The listing builds one solid part. Answer for the finished solid, in the listing's coordinates (mm). Face numbers are marked on the shaded views. A direction names the side the tool comes from. Give positions to 0.01 mm unless a question says otherwise; leave off trailing zeros. Loops run counter-clockwise (first coordinate to the right, second up) from the corner with the lowest first, then second, coordinate; pieces in that order, holes last. Notation, with made-up numbers: (20, -2) - (59, -2) arc R22 cw to (59, 15) - close; hole circle Ø11 at (52, 65.25). An arc over 180 degrees is marked (long way). Write item = value, one per line. Start each with the question number.
1) The part is cut by section D-D on x = 16.5. Write down the section's boundary in (y, z), plus the area to 3 significant figures.
2) The part is cut by section A-A on x = 0. Write down the section's boundary in (y, z).
3) The part is cut by section C-C on y = 0. Write down the section's boundary in (x, z).
4) Which of the six approach directions +Z, -Z, +X, -X, +Y, -Y give full straight-line access (tool end or side, diameter ignored) to the marked faces 1, 2 and 3?
5) Consider probe 1 along X at (y, z) = (-29, 14); probe 2 along Y at (x, z) = (15.5, 6.3); probe 3 along Y at (x, z) = (-8, 39.5). Determine where each line is inside the solid, lowest interval first.
6) The part is cut by section B-B on z = 31. Write down the section's boundary in (x, y).
7) Flat-ended cylindrical pins translate along their axes: P1, Ø10, axis at x = 2.5, z = 25.5, coming from the +Y side; P2, Ø2.5, axis at x = 8, y = -8, coming from the +Z side; P3, Ø4, axis at x = -8, y = -8, coming from the +Z side; P4, Ø3.5, axis at x = -8.5, z = 31, coming from the +Y side. Find the tip coordinate at first contact, or state that the pin passes through.
8) The mould has two halves that part along Y. Classify the marked faces 4, 5 and 6: +Y half, -Y half, draft (parallel to the pull), parting line (faces both ways), or undercut.
from build123d import *

# Parameters (mm, degrees)
MOTOR_MOUNT_SOLID_DEPTH                   = 7.5
ENCODER_DISTANCE_SKETCH_W                 = 50
ENCODER_DISTANCE_SKETCH_H                 = 45
ENCODER_DISTANCE_SOLID_DEPTH              = 5
ENCODER_MOUNT_SKETCH_R                    = 1.45
ENCODER_MOUNT_SKETCH_W                    = 7
ENCODER_MOUNT_SKETCH_H                    = 9
ENCODER_MOUNT_SOLID_DEPTH                 = 5
MOTOR_CLAMP_MOUNTING_HOLES_CUT_DEPTH      = 78.661122835
MOTOR_CLAMP_MOUNTING_HOLES_CUT_DEPTH_BACK = 78.661122835
MOTOR_CLAMP_MOUNTING_HOLES_SKETCH_R       = 1.45
GUSSET_PLATE_SKETCH_W                     = 50
GUSSET_PLATE_SKETCH_H                     = 5
GUSSET_PLATE_SOLID_DEPTH                  = 16.5
GUSSET_SOLID_DEPTH                        = 1.5
MOUNTING_PLATE_SKETCH_W                   = 50
MOUNTING_PLATE_SKETCH_H                   = 92
MOUNTING_PLATE_SKETCH_R                   = 2.65
MOUNTING_PLATE_SOLID_DEPTH                = 5
MOUNTING_HOLES_CUT_DEPTH                  = 93.348524623
MOUNTING_HOLES_CUT_DEPTH_BACK             = 93.348524623
MOUNTING_HOLE_SKETCH_R                    = 2.65
MOUNTING_PLATE_TRIM_SKETCH_W              = 50
MOUNTING_PLATE_TRIM_SKETCH_H              = 25.5
MOUNTING_PLATE_TRIM_SKETCH_H_2            = 30
MOUNTING_PLATE_TRIM_SKETCH_W_2            = 23.5
MOUNTING_PLATE_TRIM_SKETCH_H_3            = 16.5
MOUNTING_PLATE_TRIM_CUT_DEPTH             = 2
CUT_EXTRUDE1_DEPTH                        = 93.990590922
CUT_EXTRUDE1_DEPTH_BACK                   = 93.990590922
SKETCH2_W                                 = 50
SKETCH2_H                                 = 120
SKETCH2_W_2                               = 42
SKETCH2_H_2                               = 54.272597004
SKETCH3_W                                 = 42
SKETCH3_H                                 = 59.586450004
BOSS_EXTRUDE1_DEPTH                       = 5
CUT_EXTRUDE2_DEPTH                        = 69.16716098
CUT_EXTRUDE2_DEPTH_BACK                   = 69.16716098
SKETCH4_R                                 = 2.15
SKETCH5_W                                 = 42
SKETCH5_H                                 = 42
BOSS_EXTRUDE2_DEPTH                       = 5
SKETCH6_W                                 = 42
SKETCH6_H                                 = 53.136298502
CUT_EXTRUDE3_DEPTH                        = 10
SKETCH7_R                                 = 12.5
SKETCH7_R_2                               = 1.7
CUT_EXTRUDE4_DEPTH                        = 5
SKETCH8_R                                 = 5
CUT_EXTRUDE5_DEPTH                        = 56.441335495


with BuildPart() as part:
    # Mouting Mount Sketch → Motor Mount Solid (new, symmetric)
    with BuildSketch(Plane.XY):
        with BuildLine():
            Line((-25, -55), (25, -55))
            Line((25, -55), (25, 0))
            Line((25, 0), (10, 0))
            ThreePointArc((10, 0), (0, -10), (-10, 0))
            Line((-10, 0), (-25, 0))
            Line((-25, 0), (-25, -55))
        make_face()
    extrude(amount=MOTOR_MOUNT_SOLID_DEPTH, both=True)

    # Encoder Distance Sketch → Encoder Distance Solid (add)
    with BuildSketch(Plane.XZ.offset(55)):
        with Locations((0, 15)):
            Rectangle(ENCODER_DISTANCE_SKETCH_W, ENCODER_DISTANCE_SKETCH_H)
    extrude(amount=ENCODER_DISTANCE_SOLID_DEPTH)

    # Encoder Mount Sketch → Encoder Mount Solid (add)
    with BuildSketch(Plane.XY.offset(37.5)):
        Polygon((-25, -60), (-25, -55), (-11.5, 11.5), (11.5, 11.5), (25, -55), (25, -60), align=None)
        with Locations((-8, 8)):
            Circle(ENCODER_MOUNT_SKETCH_R, mode=Mode.SUBTRACT)
        with Locations((8, 8)):
            Circle(ENCODER_MOUNT_SKETCH_R, mode=Mode.SUBTRACT)
        with Locations((-8, -8)):
            Circle(ENCODER_MOUNT_SKETCH_R, mode=Mode.SUBTRACT)
        with Locations((8, -8)):
            Circle(ENCODER_MOUNT_SKETCH_R, mode=Mode.SUBTRACT)
        with Locations((-8, 0)):
            Rectangle(ENCODER_MOUNT_SKETCH_W, ENCODER_MOUNT_SKETCH_H, mode=Mode.SUBTRACT)
        with Locations((8, 0)):
            Rectangle(ENCODER_MOUNT_SKETCH_W, ENCODER_MOUNT_SKETCH_H, mode=Mode.SUBTRACT)
    extrude(amount=ENCODER_MOUNT_SOLID_DEPTH)

    # Motor Clamp Mounting Holes Sketch → Motor Clamp Mounting Holes Cut (cut, two sides: drawn at the far end of the back side and taken through both)
    with BuildSketch(Plane(origin=(0, 0, 0), x_dir=(1, 0, 0), z_dir=(0, 1, 0)).offset(-MOTOR_CLAMP_MOUNTING_HOLES_CUT_DEPTH_BACK)):
        with Locations(Location((-15, 0, 0), (0, 0, 180))):
            Circle(MOTOR_CLAMP_MOUNTING_HOLES_SKETCH_R)
        with Locations(Location((15, 0, 0), (0, 0, 180))):
            Circle(MOTOR_CLAMP_MOUNTING_HOLES_SKETCH_R)
    extrude(amount=MOTOR_CLAMP_MOUNTING_HOLES_CUT_DEPTH + MOTOR_CLAMP_MOUNTING_HOLES_CUT_DEPTH_BACK, mode=Mode.SUBTRACT)

    # Gusset Plate Sketch → Gusset Plate Solid (add)
    with BuildSketch(Plane.XY.offset(42.5)):
        with Locations((0, -57.5)):
            Rectangle(GUSSET_PLATE_SKETCH_W, GUSSET_PLATE_SKETCH_H)
    extrude(amount=GUSSET_PLATE_SOLID_DEPTH)

    # Gusset Sketch → Gusset Solid (add, symmetric)
    with BuildSketch(Plane(origin=(0, 0, 0), x_dir=(0, 0, -1), z_dir=(1, 0, 0))):
        Polygon((-42.5, 11.5), (-59, -55), (-42.5, -55), align=None)
    extrude(amount=GUSSET_SOLID_DEPTH, both=True)

    # Mounting Plate Sketch → Mounting Plate Solid (add)
    with BuildSketch(Plane(origin=(0, -55, 0), x_dir=(1, 0, 0), z_dir=(0, 1, 0))):
        with Locations((0, -13)):
            Rectangle(MOUNTING_PLATE_SKETCH_W, MOUNTING_PLATE_SKETCH_H)
        with Locations((-19, -53)):
            Circle(MOUNTING_PLATE_SKETCH_R, mode=Mode.SUBTRACT)
        with Locations((19, -53)):
            Circle(MOUNTING_PLATE_SKETCH_R, mode=Mode.SUBTRACT)
        with Locations(Location((-19, 27, 0), (0, 0, 270))):
            Circle(MOUNTING_PLATE_SKETCH_R, mode=Mode.SUBTRACT)
        with Locations(Location((19, 27, 0), (0, 0, 270))):
            Circle(MOUNTING_PLATE_SKETCH_R, mode=Mode.SUBTRACT)
    extrude(amount=-MOUNTING_PLATE_SOLID_DEPTH)

    # Mounting Hole Sketch → Mounting Holes Cut (cut, two sides: drawn at the far end of the back side and taken through both)
    with BuildSketch(Plane(origin=(0, -55, 0), x_dir=(1, 0, 0), z_dir=(0, 1, 0)).offset(-MOUNTING_HOLES_CUT_DEPTH_BACK)):
        with Locations(Location((-19, 27, 0), (0, 0, 270))):
            Circle(MOUNTING_HOLE_SKETCH_R)
        with Locations(Location((19, 27, 0), (0, 0, 270))):
            Circle(MOUNTING_HOLE_SKETCH_R)
        with Locations(Location((19, -53, 0), (0, 0, 90))):
            Circle(MOUNTING_HOLE_SKETCH_R)
        with Locations(Location((-19, -53, 0), (0, 0, 90))):
            Circle(MOUNTING_HOLE_SKETCH_R)
    extrude(amount=MOUNTING_HOLES_CUT_DEPTH + MOUNTING_HOLES_CUT_DEPTH_BACK, mode=Mode.SUBTRACT)

    # Mounting Plate Trim Sketch → Mounting Plate Trim Cut (cut)
    with BuildSketch(Plane(origin=(0, -55, 0), x_dir=(1, 0, 0), z_dir=(0, 1, 0))):
        with Locations((0, 20.25)):
            Rectangle(MOUNTING_PLATE_TRIM_SKETCH_W, MOUNTING_PLATE_TRIM_SKETCH_H)
        with Locations((0, -22.5)):
            Rectangle(MOUNTING_PLATE_TRIM_SKETCH_W, MOUNTING_PLATE_TRIM_SKETCH_H_2)
        with Locations((13.25, -50.75)):
            Rectangle(MOUNTING_PLATE_TRIM_SKETCH_W_2, MOUNTING_PLATE_TRIM_SKETCH_H_3)
        with Locations((-13.25, -50.75)):
            Rectangle(MOUNTING_PLATE_TRIM_SKETCH_W_2, MOUNTING_PLATE_TRIM_SKETCH_H_3)
    extrude(amount=-MOUNTING_PLATE_TRIM_CUT_DEPTH, mode=Mode.SUBTRACT)

    # Sketch2 → Cut-Extrude1 (cut, two sides: drawn at the far end of the back side and taken through both)
    with BuildSketch(Plane(origin=(0, 0, -7.5), x_dir=(-1, 0, 0), z_dir=(0, 0, -1)).offset(-CUT_EXTRUDE1_DEPTH_BACK)):
        Rectangle(SKETCH2_W, SKETCH2_H)
        Rectangle(SKETCH2_W_2, SKETCH2_H_2, mode=Mode.SUBTRACT)
    extrude(amount=CUT_EXTRUDE1_DEPTH + CUT_EXTRUDE1_DEPTH_BACK, mode=Mode.SUBTRACT)


with BuildPart() as cut_extrude1_piece_1:
    # of the separate pieces the step leaves, piece 1, a body of its own (cut_extrude1_pieces)
    add(part.part.solids().sort_by_distance((21, 0, 7.5))[0])



with BuildPart() as cut_extrude1_piece_2:
    # of the separate pieces the step leaves, piece 2, a body of its own (cut_extrude1_pieces)
    add(part.part.solids().sort_by_distance((-1.5, -27.136298502, 42.5))[0])


with BuildPart() as cut_extrude1_piece_1_1:
    add(cut_extrude1_piece_1.part)

    add(cut_extrude1_piece_2.part)  # Boss-Extrude1 merges Cut-Extrude1 piece 2
    # Sketch3 → Boss-Extrude1 (add)
    with BuildSketch(Plane.XZ.offset(27.136298502)):
        with Locations((0, 22.293225002)):
            Rectangle(SKETCH3_W, SKETCH3_H)
    extrude(amount=BOSS_EXTRUDE1_DEPTH)

    # Sketch4 → Cut-Extrude2 (cut, two sides: drawn at the far end of the back side and taken through both)
    with BuildSketch(Plane(origin=(0, -27.136298502, 0), x_dir=(1, 0, 0), z_dir=(0, 1, 0)).offset(-CUT_EXTRUDE2_DEPTH_BACK)):
        with Locations(Location((-8.5, -14, 0), (0, 0, 270))):
            Circle(SKETCH4_R)
        with Locations(Location((8.5, -14, 0), (0, 0, 270))):
            Circle(SKETCH4_R)
        with Locations(Location((-8.5, -31, 0), (0, 0, 270))):
            Circle(SKETCH4_R)
        with Locations(Location((8.5, -31, 0), (0, 0, 270))):
            Circle(SKETCH4_R)
    extrude(amount=CUT_EXTRUDE2_DEPTH + CUT_EXTRUDE2_DEPTH_BACK, mode=Mode.SUBTRACT)

    # Sketch5 → Boss-Extrude2 (add)
    with BuildSketch(Plane.XY.offset(7.5)):
        Rectangle(SKETCH5_W, SKETCH5_H)
    extrude(amount=-BOSS_EXTRUDE2_DEPTH)

    # Sketch6 → Cut-Extrude3 (cut)
    with BuildSketch(Plane(origin=(0, 0, -7.5), x_dir=(-1, 0, 0), z_dir=(0, 0, -1))):
        with Locations((0, -5.568149251)):
            Rectangle(SKETCH6_W, SKETCH6_H)
    extrude(amount=-CUT_EXTRUDE3_DEPTH, mode=Mode.SUBTRACT)

    # Sketch7 → Cut-Extrude4 (cut)
    with BuildSketch(Plane(origin=(0, 0, 2.5), x_dir=(-1, 0, 0), z_dir=(0, 0, -1))):
        Circle(SKETCH7_R)
        with Locations((-15.5, 15.5)):
            Circle(SKETCH7_R_2)
        with Locations((15.5, 15.5)):
            Circle(SKETCH7_R_2)
        with Locations((-15.5, -15.5)):
            Circle(SKETCH7_R_2)
        with Locations((15.5, -15.5)):
            Circle(SKETCH7_R_2)
    extrude(amount=-CUT_EXTRUDE4_DEPTH, mode=Mode.SUBTRACT)

    # Sketch8 → Cut-Extrude5 (cut, through all)
    with BuildSketch(Plane.XY.offset(42.5)):
        with Locations((-6.5, -22.136298502)):
            Circle(SKETCH8_R)
        with Locations((6.5, -22.136298502)):
            Circle(SKETCH8_R)
    extrude(amount=-CUT_EXTRUDE5_DEPTH, mode=Mode.SUBTRACT)


solid = cut_extrude1_piece_1_1.part
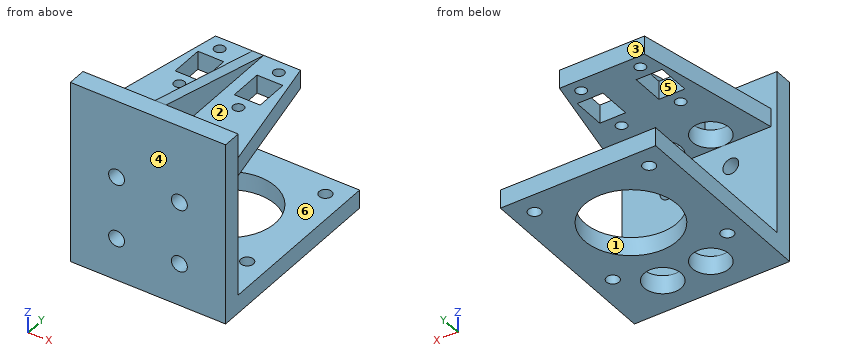
Answer below:
q1.outline = (-32.14, 2.5) - (-16.87, 2.5) - (-16.87, 7.5) - (-27.14, 7.5) - (-27.14, 37.5) - (-13.13, 37.5) - (-13.13, 42.5) - (-27.14, 42.5) - (-27.14, 52.09) - (-32.14, 52.09) - close; (-14.13, 2.5) - (14.13, 2.5) - (14.13, 7.5) - (-14.13, 7.5) - close; (16.87, 2.5) - (21, 2.5) - (21, 7.5) - (16.87, 7.5) - close
q1.area = 531 mm2
q2.outline = (-32.14, 2.5) - (-12.5, 2.5) - (-12.5, 7.5) - (-27.14, 7.5) - (-27.14, 37.5) - (11.5, 37.5) - (11.5, 42.5) - (-27.14, 52.09) - (-32.14, 52.09) - close; (12.5, 2.5) - (21, 2.5) - (21, 7.5) - (12.5, 7.5) - close
q3.outline = (-21, 2.5) - (-12.5, 2.5) - (-12.5, 7.5) - (-21, 7.5) - close; (-13.83, 37.5) - (-11.5, 37.5) - (-11.5, 42.5) - (-13.83, 42.5) - close; (-4.5, 37.5) - (4.5, 37.5) - (4.5, 42.5) - (1.5, 42.5) - (1.5, 45.35) - (-1.5, 45.35) - (-1.5, 42.5) - (-4.5, 42.5) - close; (11.5, 37.5) - (13.83, 37.5) - (13.83, 42.5) - (11.5, 42.5) - close; (12.5, 2.5) - (21, 2.5) - (21, 7.5) - (12.5, 7.5) - close
q4.face_1 = -Z
q4.face_2 = +Z, +X, +Y
q4.face_3 = +Z, +X, -X, +Y
q5.probe_1 = -21 to -10.65, -6.35 to 6.35, 10.65 to 21
q5.probe_2 = -32.14 to -17.2, -13.8 to 13.8, 17.2 to 21
q5.probe_3 = -32.14 to -26.91, -17.37 to -9.45, -6.55 to -4.5, 4.5 to 6.55, 9.45 to 11.5
q6.outline = (-21, -32.14) - (-10.65, -32.14) - (-10.65, -27.14) - (-21, -27.14) - close; (-6.35, -32.14) - (6.35, -32.14) - (6.35, -27.14) - (-6.35, -27.14) - close; (10.65, -32.14) - (21, -32.14) - (21, -27.14) - (10.65, -27.14) - close
q7.P1 = -27.14
q7.P2 = 7.5
q7.P3 = 42.5
q7.P4 = through
q8.face_4 = -Y half
q8.face_5 = undercut
q8.face_6 = draft
